Can you work these out from the drawing? Everything is in mm from the part's minimum corner. A direction names the side the tool comes from. Coordinates: 2 decimals unless noted, no trailing zeros. Loops run counter-clockwise (first coordinate to the right, second up) from the corner with the lowest first, then second, coordinate; pieces in that order, holes last. Notation, with made-up numbers: (11, -27.5) -> (38, -27.5) arc R19 ccw to (38, 9.5) -> close; hole circle Ø1 at (-27, -19.5). An arc over 180 degrees is marked (long way). Use one line per item in the form item = value. Start each with the question number.
(1) On a 3-axis mill with a long thin cutter (end or side, diameter ignored), from which of +Z, -Z, +X, -X, +Y, -Y can I reach the whole of each face in a straight line? I mean the marked faces 4 and 5. Say none if no direction works.
(2) Imagine slicing it at C-C (z = 7). List the corners of the cut face in (x, y) for me (3 decimals), plus the area to 3 significant figures.
(3) I need wall thicknesses on line 1 (Y direction, x = 6.5, z = 6) (3 decimals); line 2 (Z direction, x = 12, y = 3.25); line 3 (Y direction, x = 6, z = 1). Which ranges of each line are inside material? Lowest first, please. Write a range as [from, to].
(4) Imagine slicing it at B-B (x = 6.5). List the corners of the cut face in (y, z) for me (3 decimals).
(5) Imagine slicing it at A-A (y = 6.5). List the corners of the cut face in (x, z) for me (3 decimals).
(6) Thinking about a two-plate mould opening in Y: for the marked faces 1, 2 and 3, which applies, released by +Y, released by -Y, zero draft, split by the parting line, or undercut?
(7) Imagine slicing it at D-D (y = 12.25). List the corners of the cut face in (x, z) for me, plus the area to 3 significant figures.
(8) I'm going to push flat-ended pins straight in: pin 1 (5 mm diameter, centred on y = 6.5, z = 6.5, fed in from +X); pin 2 (5.5 mm diameter, centred on x = 6.5, y = 6.5, fed in from +Z); pin 3 (4 mm diameter, centred on x = 2.5, z = 4.5, fed in from +Y); pin 4 (4 mm diameter, centred on y = 5, z = 7, fed in from +X). Where does each tip first touch, or does it pass through?
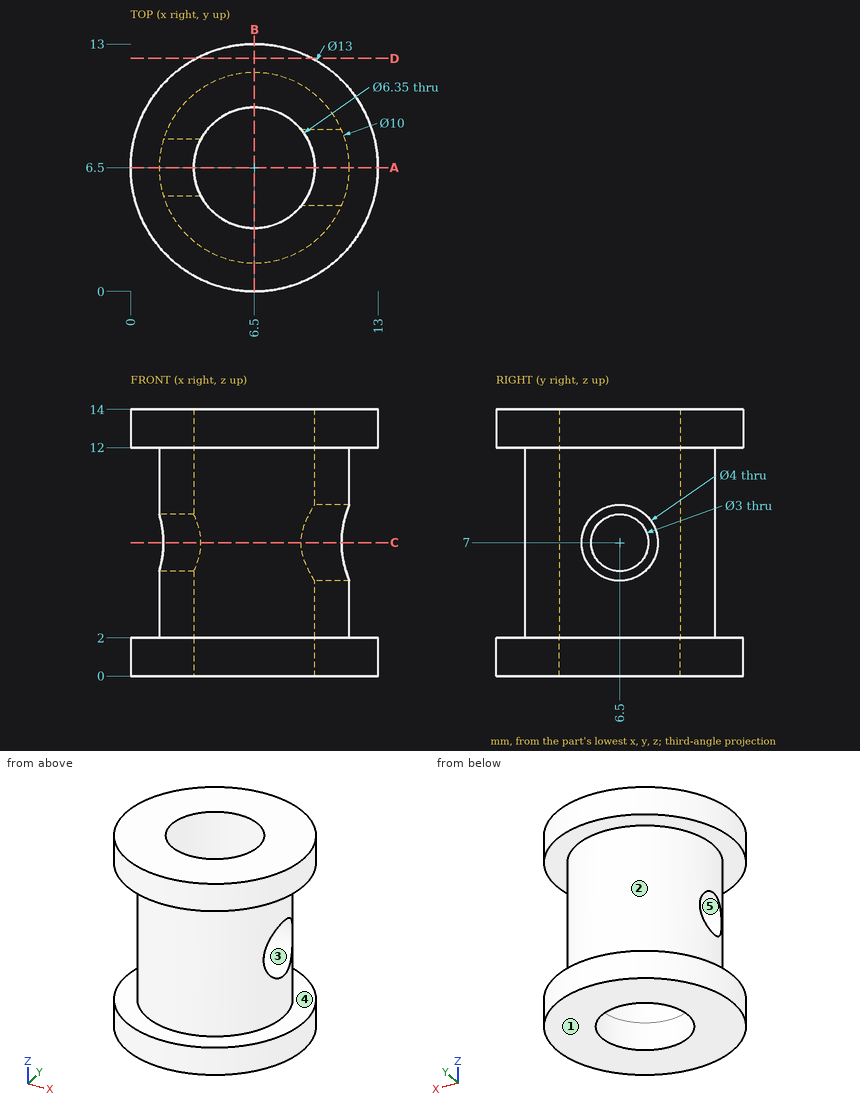
Worked out:
q1.face_4 = none
q1.face_5 = +X, -X
q2.outline = (1.73, 5) arc R5 ccw to (11.083, 4.5) -> (8.966, 4.5) arc R3.175 cw to (3.702, 5) -> close; (1.73, 8) -> (3.702, 8) arc R3.175 cw to (8.966, 8.5) -> (11.083, 8.5) arc R5 ccw to start
q2.area = 33.6 mm2
q3.line_1 = [1.5, 3.325], [9.675, 11.5]
q3.line_2 = [0, 2], [12, 14]
q3.line_3 = [0.02, 3.36], [9.64, 12.98]
q4.outline = (0, 0) -> (3.325, 0) -> (3.325, 14) -> (0, 14) -> (0, 12) -> (1.5, 12) -> (1.5, 2) -> (0, 2) -> close; (9.675, 0) -> (13, 0) -> (13, 2) -> (11.5, 2) -> (11.5, 12) -> (13, 12) -> (13, 14) -> (9.675, 14) -> close
q5.outline = (0, 0) -> (3.325, 0) -> (3.325, 5.5) -> (1.5, 5.5) -> (1.5, 2) -> (0, 2) -> close; (0, 12) -> (1.5, 12) -> (1.5, 8.5) -> (3.325, 8.5) -> (3.325, 14) -> (0, 14) -> close; (9.675, 0) -> (13, 0) -> (13, 2) -> (11.5, 2) -> (11.5, 5) -> (9.675, 5) -> close; (9.675, 9) -> (11.5, 9) -> (11.5, 12) -> (13, 12) -> (13, 14) -> (9.675, 14) -> close
q6.face_1 = zero draft
q6.face_2 = split by the parting line
q6.face_3 = undercut
q7.outline = (3.47, 0) -> (9.53, 0) -> (9.53, 2) -> (3.47, 2) -> close; (3.47, 12) -> (9.53, 12) -> (9.53, 14) -> (3.47, 14) -> close
q7.area = 24.2 mm2
q8.pin_1 = 11.5
q8.pin_2 = through
q8.pin_3 = 11.08
q8.pin_4 = 11.44
